Here's how the part is built. I have some questions about the finished solid (model axes, mm). A direction names the side the tool comes from. Round coordinates to 2 decimals unless told otherwise and drop trailing zeros. Order: outer loops, then holes, each group sorted by start corner. A loop starts at its lowest first (then second) coordinate and runs counter-clockwise, first axis right, second up. Notation, with made-up numbers: (54, 23) -> (74, 23) arc R31 ccw to (74, 57) -> close; hole circle Ø1 at (12, 86). An arc over 180 degrees is marked (long way). One line per item, written item: value.
```python
from build123d import *

# Parameters (mm, degrees)
SKETCH1_W               = 161
SKETCH1_H               = 15
BOSS_EXTRUDE1_DEPTH     = 4
SKETCH2_W               = 3
SKETCH2_H               = 15
BOSS_EXTRUDE2_DEPTH     = 20
SKETCH4_R               = 1.8
CUT_EXTRUDE2_DEPTH      = 1
CUT_EXTRUDE2_DEPTH_BACK = 162
BOSS_EXTRUDE3_DEPTH     = 19


with BuildPart() as part:
    # Sketch1 → Boss-Extrude1 (new body)
    with BuildSketch(Plane(origin=(0, 0, 0), x_dir=(1, 0, 0), z_dir=(0, 1, 0))):
        Rectangle(SKETCH1_W, SKETCH1_H)
    extrude(amount=BOSS_EXTRUDE1_DEPTH)

    # Sketch2 → Boss-Extrude2 (add)
    with BuildSketch(Plane(origin=(0, 4, 0), x_dir=(1, 0, 0), z_dir=(0, 1, 0))):
        with Locations((-48.5, 0)):
            Rectangle(SKETCH2_W, SKETCH2_H)
        with Locations((-79, 0)):
            Rectangle(SKETCH2_W, SKETCH2_H)
        with Locations((79, 0)):
            Rectangle(SKETCH2_W, SKETCH2_H)
        with Locations((48.5, 0)):
            Rectangle(SKETCH2_W, SKETCH2_H)
    extrude(amount=BOSS_EXTRUDE2_DEPTH)

    # Sketch4 → Cut-Extrude2 (cut, two sides)
    with BuildSketch(Plane.ZY.offset(80.5)) as cut_extrude2_sk:
        with Locations((4, 18)):
            Circle(SKETCH4_R)
        with Locations((-4, 18)):
            Circle(SKETCH4_R)
    extrude(amount=CUT_EXTRUDE2_DEPTH, mode=Mode.SUBTRACT)
    extrude(cut_extrude2_sk.sketch, amount=-CUT_EXTRUDE2_DEPTH_BACK, mode=Mode.SUBTRACT)

    # Sketch5 → Boss-Extrude3 (add)
    with BuildSketch(Plane.XZ):
        with BuildLine():
            Line((-7.75, -4.75), (7.75, -4.75))
            ThreePointArc((7.75, -4.75), (8.457106781, -4.457106781), (8.75, -3.75))
            Line((8.75, -3.75), (8.75, 3.75))
            ThreePointArc((8.75, 3.75), (8.457106781, 4.457106781), (7.75, 4.75))
            Line((7.75, 4.75), (-7.75, 4.75))
            ThreePointArc((-7.75, 4.75), (-8.457106781, 4.457106781), (-8.75, 3.75))
            Line((-8.75, 3.75), (-8.75, -3.75))
            ThreePointArc((-8.75, -3.75), (-8.457106781, -4.457106781), (-7.75, -4.75))
        make_face()
    extrude(amount=BOSS_EXTRUDE3_DEPTH)


solid = part.part
```
Q1. For P1, Ø10, axis at x = 53.5, y = -6.5, coming from the +Z side; P2, Ø2, axis at y = -11, z = 5.5, coming from the -X side; P3, Ø4.5, axis at x = -67, z = 2, coming from the +Y side; P4, Ø4.5, axis at x = 31.5, z = 3, coming from the -Y side, each with a flat end and sliding along its axis, tell me the tip position at first contact or that it passes through.
Answers:
P1: through
P2: x = -8.41
P3: y = 4
P4: y = 0
Q2. Which directions (+Z, -Z, +X, -X, +Y, -Y) give clear straight access to the entire face, cutting with the end or side of a thin tool? Please do faces 5 (the face through (50, 14, 0)), 6 (the face through (0, -9, -4.75)), 7 (the face through (0, -19, 0)), 8 (the face through (48.479, 19.785, 3.766)), 9 (the face through (-8.75, -9, 0)).
Answers:
face 5: +Z, -Z, +Y
face 6: -Z, +X, -X, -Y
face 7: +Z, -Z, +X, -X, -Y
face 8: +X, -X
face 9: +Z, -Z, -X, -Y
Q3. I want a section at A-A on y = 7. Write out the boundary of the cut face in (x, z), then the cut area to 3 significant figures.
Answers:
outline: (-80.5, -7.5) -> (-77.5, -7.5) -> (-77.5, 7.5) -> (-80.5, 7.5) -> close; (-50, -7.5) -> (-47, -7.5) -> (-47, 7.5) -> (-50, 7.5) -> close; (47, -7.5) -> (50, -7.5) -> (50, 7.5) -> (47, 7.5) -> close; (77.5, -7.5) -> (80.5, -7.5) -> (80.5, 7.5) -> (77.5, 7.5) -> close
area: 180 mm2
Q4. I want a section at B-B on x = 5. Write out the boundary of the cut face in (y, z), then the cut area to 4 significant figures.
Answers:
outline: (-19, -4.75) -> (0, -4.75) -> (0, -7.5) -> (4, -7.5) -> (4, 7.5) -> (0, 7.5) -> (0, 4.75) -> (-19, 4.75) -> close
area: 240.5 mm2
Q5. I want a section at C-C on y = -6. Write out the boundary of the cut face in (x, z), then the cut area to 3 significant figures.
Answers:
outline: (-8.75, -3.75) arc R1 ccw to (-7.75, -4.75) -> (7.75, -4.75) arc R1 ccw to (8.75, -3.75) -> (8.75, 3.75) arc R1 ccw to (7.75, 4.75) -> (-7.75, 4.75) arc R1 ccw to (-8.75, 3.75) -> close
area: 165 mm2
Q6. I want a section at D-D on y = 18. Give the number of separate pieces and of enclosed holes in the cut face, then the cut area to 3 significant figures.
Answers:
separate pieces: 12
enclosed holes: 0
area: 93.6 mm2
Q7. If we mould it in two halves opening along Y, with no side actions, what happens to faces 1 (the face through (48, 24, 0)), 2 (the face through (48.479, 19.785, -4.234)), 3 (the face through (8.75, -9, 0)), 4 (the face through (78.979, 19.785, 3.766))? For each: pulls with the +Y half, pulls with the -Y half, needs draft (parallel to the pull), parting line crosses it, or undercut.
Answers:
face 1: pulls with the +Y half
face 2: undercut
face 3: needs draft
face 4: undercut
Q8. I need wall thicknesses on line 1 along X through (y, z) = (16, 1); line 2 along Y through (x, z) = (48, 4); line 3 along Y through (x, z) = (-73.5, -7). Which ranges of each line are inside material? Lowest first, please.
Answers:
line 1: -80.5 to -77.5, -50 to -47, 47 to 50, 77.5 to 80.5
line 2: 0 to 16.2, 19.8 to 24
line 3: 0 to 4
